Check sheet for the modelled part. Datum: model origin and axes. Units: mm. A direction names the side the tool comes from. Give positions to 0.01 mm unless a question says otherwise; leave off trailing zeros. Order: outer loops, then holes, each group sorted by start corner. A loop starts at its lowest first (then second) coordinate and runs counter-clockwise, first axis right, second up. Notation, with made-up numbers: (-10, 49.25) - (42, 49.25) arc R23 ccw to (42, 70.25) - close; hole circle Ø6 at (1.5, 30.5). An arc over 180 degrees is marked (long way). Answer in a Markdown table with one row per item.
from build123d import *

# Parameters (mm, degrees)
BASE_EXTRUDE_DEPTH = 22.987
CUT_EXTRUDE1_DEPTH = 1.524
CUT_EXTRUDE2_START = -13.3858
CUT_EXTRUDE2_DEPTH = 13.3858
CUT_EXTRUDE3_DEPTH = 11.8618
SKETCH5_R          = 8.73125
CUT_EXTRUDE4_DEPTH = 165.748162847
SKETCH6_R          = 13.97
CUT_EXTRUDE5_DEPTH = 165.9536267
CUT_EXTRUDE6_DEPTH = 165.9536267


with BuildPart() as part:
    # Sketch1 → Base-Extrude (new body)
    with BuildSketch(Plane.XY):
        with BuildLine():
            Line((67.622164121, 48.488607139), (60.451998121, 48.488607139))
            ThreePointArc((60.451998121, 48.488607139), (58.415767784, 48.225162891), (56.513628913, 47.45217869))
            Line((56.513628913, 47.45217869), (-6.63896207, 11.740278591))
            ThreePointArc((-6.63896207, 11.740278591), (-13.04330848, -3.432500932), (0, -13.4874))
            Line((0, -13.4874), (108.3963288, -13.4874))
            ThreePointArc((108.3963288, -13.4874), (116.52844195, -14.610715729), (124.051506942, -17.896533077))
            ThreePointArc((124.051506942, -17.896533077), (153.760306668, -9.394598854), (142.773406597, 19.487639521))
            Line((142.773406597, 19.487639521), (72.327100379, 47.584944713))
            ThreePointArc((72.327100379, 47.584944713), (70.017630202, 48.26064561), (67.622164121, 48.488607139))
        make_face()
    extrude(amount=BASE_EXTRUDE_DEPTH)

    # Sketch2 → Cut-Extrude1 (cut)
    with BuildSketch(Plane.XY.offset(22.987)):
        with BuildLine():
            Line((52.451, 40.561691476), (52.451, -5.6134))
            ThreePointArc((52.451, -5.6134), (54.757241386, -11.181158976), (60.325000513, -13.4874))
            Line((60.325000513, -13.4874), (60.325000513, -28.150605259))
            Line((60.325000513, -28.150605259), (-23.486257356, -28.150605259))
            Line((-23.486257356, -28.150605259), (-22.173444803, 52.159193632))
            Line((-22.173444803, 52.159193632), (56.513628913, 52.159193632))
            Line((56.513628913, 52.159193632), (56.513628913, 47.45217869))
            Line((56.513628913, 47.45217869), (56.449146437, 47.415714759))
            ThreePointArc((56.449146437, 47.415714759), (53.523590332, 44.529146898), (52.451, 40.561691476))
        make_face()
    extrude(amount=-CUT_EXTRUDE1_DEPTH, mode=Mode.SUBTRACT)

    # Sketch3 → Cut-Extrude2 (cut)
    with BuildSketch(Plane(origin=(0, 0, 0), x_dir=(-1, 0, 0), z_dir=(0, 0, -1)).offset(CUT_EXTRUDE2_START)):
        with BuildLine():
            Line((-52.451, 40.561691476), (-52.451, -5.6134))
            ThreePointArc((-52.451, -5.6134), (-54.757241386, -11.181158976), (-60.325000513, -13.4874))
            Line((-60.325000513, -13.4874), (-60.325000513, -35.585726692))
            Line((-60.325000513, -35.585726692), (18.461929403, -35.585726692))
            Line((18.461929403, -35.585726692), (18.461929403, 62.437610527))
            Line((18.461929403, 62.437610527), (-56.449146437, 62.437610527))
            Line((-56.449146437, 62.437610527), (-56.449146437, 47.415714759))
            ThreePointArc((-56.449146437, 47.415714759), (-53.523590332, 44.529146898), (-52.451, 40.561691476))
        make_face()
    extrude(amount=CUT_EXTRUDE2_DEPTH, mode=Mode.SUBTRACT)

    # Sketch4 → Cut-Extrude3 (cut)
    with BuildSketch(Plane(origin=(0, 0, 0), x_dir=(-1, 0, 0), z_dir=(0, 0, -1))):
        with BuildLine():
            Line((-113.4872, -5.6134), (-113.4872, 25.831689784))
            ThreePointArc((-113.4872, 25.831689784), (-112.131206016, 30.249321907), (-108.530259798, 33.145419212))
            Line((-108.530259798, 33.145419212), (-119.346107198, 60.263197686))
            Line((-119.346107198, 60.263197686), (-162.925004358, 60.263197686))
            Line((-162.925004358, 60.263197686), (-162.925004358, -25.739632552))
            Line((-162.925004358, -25.739632552), (-105.6132, -25.739632552))
            Line((-105.6132, -25.739632552), (-105.6132, -13.4874))
            ThreePointArc((-105.6132, -13.4874), (-111.180958795, -11.181158795), (-113.4872, -5.6134))
        make_face()
    extrude(amount=-CUT_EXTRUDE3_DEPTH, mode=Mode.SUBTRACT)

    # Sketch5 → Cut-Extrude4 (cut, through all)
    with BuildSketch(Plane.XY.offset(21.463)):
        Circle(SKETCH5_R)
    extrude(amount=-CUT_EXTRUDE4_DEPTH, mode=Mode.SUBTRACT)

    # Sketch6 → Cut-Extrude5 (cut, through all)
    with BuildSketch(Plane.XY.offset(22.987)):
        with Locations((135.000853225, 8.827e-05)):
            Circle(SKETCH6_R)
    extrude(amount=-CUT_EXTRUDE5_DEPTH, mode=Mode.SUBTRACT)

    # Sketch7 → Cut-Extrude6 (cut, through all)
    with BuildSketch(Plane.XY.offset(22.987)):
        with BuildLine():
            Line((64.4525, -5.4356), (64.4525, 6.5024))
            ThreePointArc((64.4525, 6.5024), (60.452, 10.5029), (56.4515, 6.5024))
            Line((56.4515, 6.5024), (56.4515, -5.4356))
            ThreePointArc((56.4515, -5.4356), (60.452, -9.4361), (64.4525, -5.4356))
        make_face()
        with BuildLine():
            Line((64.4525, 24.5618), (64.4525, 36.4998))
            ThreePointArc((64.4525, 36.4998), (60.452, 40.5003), (56.4515, 36.4998))
            Line((56.4515, 36.4998), (56.4515, 24.5618))
            ThreePointArc((56.4515, 24.5618), (60.452, 20.5613), (64.4525, 24.5618))
        make_face()
        with BuildLine():
            Line((101.4603, 10.9982), (101.4603, -0.9398))
            ThreePointArc((101.4603, -0.9398), (105.4608, -4.9403), (109.4613, -0.9398))
            Line((109.4613, -0.9398), (109.4613, 10.9982))
            ThreePointArc((109.4613, 10.9982), (105.4608, 14.9987), (101.4603, 10.9982))
        make_face()
        with BuildLine():
            Line((73.533, 29.5402), (92.456, 29.5402))
            ThreePointArc((92.456, 29.5402), (95.150076836, 28.424276836), (96.266, 25.7302))
            Line((96.266, 25.7302), (96.266, 13.2588))
            ThreePointArc((96.266, 13.2588), (95.150076836, 10.564723164), (92.456, 9.4488))
            Line((92.456, 9.4488), (73.533, 9.4488))
            ThreePointArc((73.533, 9.4488), (70.838923164, 10.564723164), (69.723, 13.2588))
            Line((69.723, 13.2588), (69.723, 25.7302))
            ThreePointArc((69.723, 25.7302), (70.838923164, 28.424276836), (73.533, 29.5402))
        make_face()
    extrude(amount=-CUT_EXTRUDE6_DEPTH, mode=Mode.SUBTRACT)


solid = part.part
(1) Access from +Z, -Z, +X, -X, +Y, -Y to the whole of each face (thin tool, end or side, straight path). Record for faces 1 (the cylindrical face through (58.44, 48.23, 11.33)), 2 (the flat face through (109.461, 5, 12)), 3 (the cylindrical face through (54.696, -11.12, 22.236)), 4 (the flat face through (52.451, 18, 7)), 5 (the cylindrical face through (111.12, -11.24, 5.85)).
Geometry says:
| item | result |
|---|---|
| face 1 | +Z, -Z, -X, +Y |
| face 2 | +Z, -Z |
| face 3 | +Z, -X, -Y |
| face 4 | -Z, -X, +Y, -Y |
| face 5 | -Z, +X, -Y |
(2) Cross-section at B-B, the plane z = 16.5. Give the number of separate pieces and of enclosed holes in the cut face, then the cut area to 3 significant figures.
Geometry says:
| item | result |
|---|---|
| separate pieces | 1 |
| enclosed holes | 6 |
| area | 5,830 mm² |
(3) Cross-section at D-D, the plane x = 36. Record the cut outline in (y, z).
Geometry says:
| item | result |
|---|---|
| outline | (-13.49, 13.39) - (35.85, 13.39) - (35.85, 21.46) - (-13.49, 21.46) - close |
(4) Cross-section at C-C, the plane y = 23. Record the cut outline in (x, z).
Geometry says:
| item | result |
|---|---|
| outline | (13.27, 13.39) - (52.45, 13.39) - (52.45, 0) - (56.77, 0) - (56.77, 22.99) - (52.45, 22.99) - (52.45, 21.46) - (13.27, 21.46) - close; (64.14, 0) - (69.72, 0) - (69.72, 22.99) - (64.14, 22.99) - close; (96.27, 0) - (113.49, 0) - (113.49, 11.86) - (133.97, 11.86) - (133.97, 22.99) - (96.27, 22.99) - close |
(5) Mould release check, pull along X, two halves, no side actions. Record for faces 6 (the cylindrical face through (112.17, 30.19, 5.85)), 7 (the flat face through (96.266, 20, 12)), 8 (the cylindrical face through (53.553, 44.579, 22.236)): pulls with the +X half, pulls with the -X half, needs draft (parallel to the pull), parting line crosses it, or undercut.
Geometry says:
| item | result |
|---|---|
| face 6 | pulls with the +X half |
| face 7 | undercut |
| face 8 | pulls with the -X half |
(6) Thickness scan on L1, parallel to X at y = 2, z = 8.5; L2, parallel to X at y = 26, z = 8; L3, parallel to Y at x = 0, z = 17. Record the ranges inside material, lowest first.
Geometry says:
| item | result |
|---|---|
| L1 | 52.45 to 56.45, 64.45 to 101.46, 109.46 to 113.49 |
| L2 | 52.45 to 56.45, 64.45 to 69.73, 96.26 to 113.49 |
| L3 | -13.49 to -8.73, 8.73 to 15.49 |
(7) Cross-section at A-A, the plane y = 3. Record the cut outline in (x, z).
Geometry says:
| item | result |
|---|---|
| outline | (-13.15, 13.39) - (-8.2, 13.39) - (-8.2, 21.46) - (-13.15, 21.46) - close; (8.2, 13.39) - (52.45, 13.39) - (52.45, 0) - (56.45, 0) - (56.45, 22.99) - (52.45, 22.99) - (52.45, 21.46) - (8.2, 21.46) - close; (64.45, 0) - (101.46, 0) - (101.46, 22.99) - (64.45, 22.99) - close; (109.46, 0) - (113.49, 0) - (113.49, 11.86) - (121.36, 11.86) - (121.36, 22.99) - (109.46, 22.99) - close; (148.64, 11.86) - (155.77, 11.86) - (155.77, 22.99) - (148.64, 22.99) - close |
(8) Gauge pin test, flat ends, axial feed: P1, Ø1, axis at x = 107.5, z = 15.5, coming from the +Y side; P2, Ø7, axis at x = 66, z = 9.5, coming from the -Y side; P3, Ø3.5, axis at y = 31, z = 7.5, coming from the +X side; P4, Ø10.5, axis at x = 0, y = 0, coming from the -Z side. Record the tip position at first contact, or that the pin passes through.
Geometry says:
| item | result |
|---|---|
| P1 | y = 33.76 |
| P2 | y = -13.49 |
| P3 | x = 112.71 |
| P4 | through |
